from build123d import *

# Parameters (mm, degrees)
BOSS_EXTRUDE1_DEPTH = 5.15
SKETCH2_R           = 1.9675
SKETCH2_W           = 4.95
SKETCH2_H           = 3.8
CUT_EXTRUDE1_DEPTH  = 6.15


with BuildPart() as part:
    # Sketch1 → Boss-Extrude1 (new body)
    with BuildSketch(Plane.XY):
        with BuildLine():
            Line((-32.057735027, 87.9), (32.057735027, 87.9))
            Line((32.057735027, 87.9), (33.694332379, 90.734669766))
            Line((33.694332379, 90.734669766), (38.154363209, 88.159669766))
            Line((38.154363209, 88.159669766), (39.912093048, 91.204147153))
            Line((39.912093048, 91.204147153), (35.452062218, 93.779147153))
            Line((35.452062218, 93.779147153), (37.009792057, 96.477214379))
            Line((37.009792057, 96.477214379), (41.469822887, 93.902214379))
            Line((41.469822887, 93.902214379), (43.227552726, 96.946691766))
            Line((43.227552726, 96.946691766), (38.767521896, 99.521691766))
            Line((38.767521896, 99.521691766), (40.433263841, 102.406841447))
            ThreePointArc((40.433263841, 102.406841447), (0, 110.1), (-40.433263841, 102.406841447))
            Line((-40.433263841, 102.406841447), (-38.767521896, 99.521691766))
            Line((-38.767521896, 99.521691766), (-43.227552726, 96.946691766))
            Line((-43.227552726, 96.946691766), (-41.469822887, 93.902214379))
            Line((-41.469822887, 93.902214379), (-37.009792057, 96.477214379))
            Line((-37.009792057, 96.477214379), (-35.452062218, 93.779147153))
            Line((-35.452062218, 93.779147153), (-39.912093048, 91.204147153))
            Line((-39.912093048, 91.204147153), (-38.154363209, 88.159669766))
            Line((-38.154363209, 88.159669766), (-33.694332379, 90.734669766))
            Line((-33.694332379, 90.734669766), (-32.057735027, 87.9))
        make_face()
    extrude(amount=BOSS_EXTRUDE1_DEPTH)

    # Sketch2 → Cut-Extrude1 (cut, through all)
    with BuildSketch(Plane.XY.offset(5.15)):
        with Locations((10.74, 104.550558367)):
            Circle(SKETCH2_R)
        with Locations((17.786830638, 104.550558367)):
            Rectangle(SKETCH2_W, SKETCH2_H)
        with Locations((3.693169362, 104.550558367)):
            Rectangle(SKETCH2_W, SKETCH2_H)
    extrude(amount=-CUT_EXTRUDE1_DEPTH, mode=Mode.SUBTRACT)


solid = part.part
Geometry: final body of the model. Coordinates: model frame, mm. A direction names the side the tool comes from. Give positions to 0.01 mm unless a question says otherwise; leave off trailing zeros. Loops run counter-clockwise (first coordinate to the right, second up) from the corner with the lowest first, then second, coordinate; pieces in that order, holes last. Notation, with made-up numbers: (12.25, 3) - (71.25, 3) arc R19 cw to (71.25, 25) - close; hole circle Ø7 at (44.5, 33.25). An arc over 180 degrees is marked (long way). Answer as CSV lines item,"result". Start each with the question number.
1. Pin query (flat end, axial travel): P1, Ø1, axis at y = 102, z = 3, coming from the -X side. Return the tip coordinate at first contact, or that it passes through.
2. Ray query, L1, parallel to X at y = 90, z = 4.9; L2, parallel to X at y = 89, z = 4.9; L3, parallel to Y at x = 10.74, z = 3.5. Return the intervals inside material, ascending.
3. Section B-B, the plane z = 4.35. Give the number of separate pieces and of enclosed holes in the cut face, plus the area to 3 significant figures.
4. Draft query along Y for faces 1 (the face through (-1, 97, 5.15)), 2 (the face through (-32.89, 89.34, 2.54)), 3 (the face through (37.713, 92.474, 2.539)). Return one class per face: released by +Y, released by -Y, zero draft, split by the parting line, or undercut.
5. Reachability of faces 4 (the face through (35.893, 89.465, 2.539)), 5 (the face through (-42.361, 95.446, 2.539)), 6 (the face through (39.589, 100.944, 2.539)), 7 (the face through (36.22, 95.11, 2.54)) from +Z, -Z, +X, -X, +Y, -Y: full face, straight path, thin tool, end or side. Return the list, or none.
6. Section C-C, the plane y = 98. Return loops of the section in (x, z).
7. Section A-A, the plane x = 10.74. Return loops of the section in (y, z).
8. Section D-D, the plane x = 23. Return loops of the section in (y, z).
Answers:
1,P1,"stops at x = -40.43"
2,L1,"x = -39.22 to -34.97, -33.27 to 33.27, 34.97 to 39.22"
2,L2,"x = -38.64 to -36.7, -32.69 to 32.69, 36.7 to 38.64"
2,L3,"y = 87.9 to 102.58, 106.52 to 109.57"
3,separate pieces,"1"
3,enclosed holes,"3"
3,area,"1,490 mm2"
4,face 1,"zero draft"
4,face 2,"released by -Y"
4,face 3,"undercut"
5,face 4,"+Z, -Z, -Y"
5,face 5,"+Z, -Z, -X, -Y"
5,face 6,"+Z, -Z, +X"
5,face 7,"+Z, -Z"
6,outline,"(-41.4, 0) - (41.4, 0) - (41.4, 5.15) - (-41.4, 5.15) - close"
7,outline,"(87.9, 0) - (102.58, 0) - (102.58, 5.15) - (87.9, 5.15) - close; (106.52, 0) - (109.57, 0) - (109.57, 5.15) - (106.52, 5.15) - close"
8,outline,"(87.9, 0) - (107.67, 0) - (107.67, 5.15) - (87.9, 5.15) - close"
